Geometry check sheet. Reference: the model listing, model coordinates, mm. Face numbers are marked on the shaded views. A direction names the side the tool comes from. Round coordinates to 2 decimals unless told otherwise and drop trailing zeros. Write each loop counter-clockwise with the first axis right and the second up, starting at its lowest first coordinate (ties: lowest second). Pieces come first, ordered by that corner, then holes. Notation, with made-up numbers: M -11,38.25 L 10,38.25 A22 ccw 10,60.25 Z; hole C -22.5,-3.5 d8. An arc over 180 degrees is marked long. One line per item, written item: value. Start each with the question number.
1. Scan lines: probe 1 along Y at (x, z) = (2.5, -4.5); probe 2 along X at (y, z) = (7.25, 0); probe 3 along X at (y, z) = (21, 1). Record each from-to range of solid material in increasing order. Write a range as [from, to].
2. Access from +Z, -Z, +X, -X, +Y, -Y to the whole of each face (thin tool, end or side, straight path). Record for the marked faces 4, 5 and 6.
3. Section check C-C (z = -4.75). Record the boundary of the cut face in (x, y), and give its area (3 significant figures).
4. Release check for a two-part mould opening along X. For the marked faces 1, 2 and 3 record: pulls with the +X half, pulls with the -X half, needs draft (parallel to the pull), parting line crosses it, or undercut.
5. Section check B-B (x = 6). Record the boundary of the cut face in (y, z), and give its area (3 significant figures).
6. Depth check by flat-ended pin: P1, Ø4, axis at y = 17, z = -3.5, coming from the +X side; P2, Ø10, axis at x = 4, y = 8, coming from the +Z side; P3, Ø6, axis at x = 10.5, y = 8, coming from the +Z side. Enter the tip coordinate at first touch or a pass-through.
7. Section check D-D (y = 6.75). Record the boundary of the cut face in (x, z).
8. Section check A-A (x = 8.25). Record the boundary of the cut face in (y, z).
Autodesk Fusion 360 part; units mm, degrees
sketch "Sketch1" plane through (0, 0, 0) normal (0, 1, 0) x (1, 0, 0)
  line L0 (-6.9583, -4.2531) -> (13.0417, -4.2531)
  line L1 (13.0417, -4.2531) -> (13.0417, 8.7469)
  line L2 (13.0417, 8.7469) -> (-6.9583, 8.7469)
  line L3 (-6.9583, 8.7469) -> (-6.9583, -4.2531)
  line L4 (-6.9583, -4.2531) -> (1.0417, -4.2531)
  line L5 (1.0417, -4.2531) -> (1.0417, 8.7469)
  line L6 (1.0417, 8.7469) -> (-6.9583, 8.7469)
  line L7 (-6.9583, 8.7469) -> (-6.9583, -4.2531)
  dimension "d4" = 20
  dimension "d5" = 13
  dimension "d7" = 8
  dimension "d8" = 13
extrude "Extrude1" add sketch "Sketch1" along normal blind 23.5 contours L0 L2 L3 L4 L5 L6 L7
extrude "Extrude2" add sketch "Sketch1" along normal blind 3 contours L0 L1 L2 L5
sketch "Sketch2" plane through (1.0417, 0, 0) normal (1, 0, 0) x (0, 1, 0)
  line L0 (3, -8.7469) -> (23.5, -8.7469)
  line L1 (23.5, -8.7469) -> (23.5, 4.2531)
  line L2 (23.5, 4.2531) -> (3, 4.2531)
  line L3 (3, -0.2469) -> (18.5, -0.2469)
  line L4 (23.5, 4.2531) -> (18.4635, 4.2531)
  line L5 (18.4635, 4.2531) -> (18.4635, -8.7469)
  line L6 (18.4635, -8.7469) -> (23.5, -8.7469)
  line L7 (23.5, -8.7469) -> (23.5, 4.2531)
  line L8 (3, 4.2531) -> (3, -8.7469)
  dimension "d16" = 15.5
extrude "Extrude3" add sketch "Sketch2" along normal blind 12 contours L0 L1 L2 L4 L5 L6 L7
fillet "Fillet1" radius 2 1 edges at (-6.9583, 23.5, -2.2469)
fillet "Fillet2" radius 2 1 edges at (-6.9583, 0, -2.2469)
fillet "Fillet3" radius 1 1 edges at (13.0417, 18.4635, -2.2469)
fillet "Fillet4" radius 1 1 edges at (13.0417, 0, -2.2469)
sketch "Sketch3" plane through (0, 23.5, 0) normal (0, 1, 0) x (-1, 0, 0)
  line L0 (4.9583, -8.7469) -> (4.9583, 4.2531)
  line L1 (4.9583, 4.2531) -> (-13.0417, 4.2531)
  line L2 (-13.0417, 4.2531) -> (-13.0417, -8.7469)
  line L3 (-13.0417, -8.7469) -> (4.9583, -8.7469)
  line L4 (4.9583, -2.2469) -> (-13.0417, -2.2469)
  line L5 (-8.5241, 4.0524) -> (-8.5241, 0.8024)
  line L6 (-8.5417, -8.8028) -> (-8.5417, -5.5528)
  circle A0 centre (-8.5241, 0.8024) radius 1.3
  circle A1 centre (-8.5417, -5.5528) radius 1.3
  line L7 (-13.0417, 0.8028) -> (-8.5417, 0.8028)
  line L8 (-13.0417, -5.5528) -> (-8.5417, -5.5528)
  dimension "d32" = 3.25
  dimension "d33" = 3.25
  dimension "d34" = 2.6
  dimension "d35" = 2.6
  dimension "d36" = 4.5
  dimension "d37" = 4.5
hole "Hole2" at (8.5417, 23.5, 0.8028) at (8.5417, 23.5, -5.5528) direction (0, -1, 0) diameter 2.529 depth 10 tip angle 118
equation "clamp_w = 20 mm"
equation "clamp_l = 13 mm"
equation "clamp_bot_thickness = 3 mm"
equation "d4 = clamp_w"
equation "d5 = clamp_l"
equation "clamp_mid_w = 8 mm"
equation "d7 = clamp_mid_w"
equation "d8 = clamp_l"
equation "clamp_mid_thickness = deck_bed_gap + clamp_bot_thickness + clamp_top_thickness"
equation "d10 = clamp_mid_thickness"
equation "d12 = clamp_bot_thickness"
equation "clamp_top_thickness = 5 mm"
equation "deck_bed_gap = 15.5 mm"
equation "d16 = deck_bed_gap"
equation "top_clamp_depth = clamp_w - clamp_mid_w"
equation "d18 = top_clamp_depth"
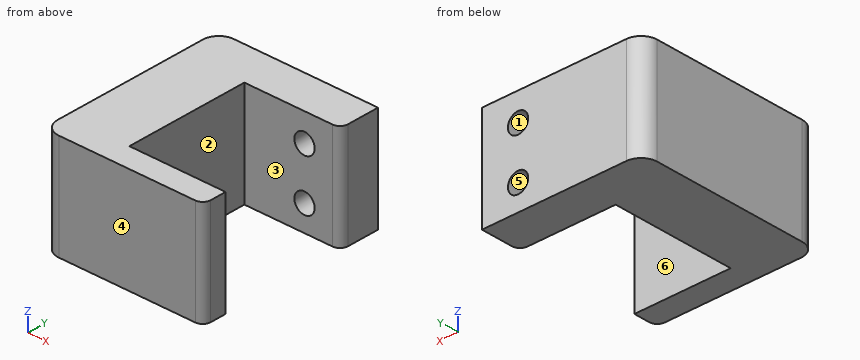
Result sheet:
1. probe 1: y = [0, 3], [18.46, 23.5]
1. probe 2: x = [-6.96, 1.04]
1. probe 3: x = [-6.96, 7.29], [9.79, 13.04]
2. face 4: +Z, -Z, +X, -X, -Y
2. face 5: +Y
2. face 6: +Z, -Z, +X
3. outline: M -6.96,2 A2 ccw -4.96,0 L 12.04,0 A1 ccw 13.04,1 L 13.04,3 L 1.04,3 L 1.04,18.46 L 7.56,18.46 L 7.56,23.5 L -4.96,23.5 A2 ccw -6.96,21.5 Z; M 9.52,18.46 L 12.04,18.46 A1 ccw 13.04,19.46 L 13.04,23.5 L 9.52,23.5 Z
3. area: 272 mm2
4. face 1: undercut
4. face 2: pulls with the +X half
4. face 3: needs draft
5. outline: M 0,-8.75 L 3,-8.75 L 3,4.25 L 0,4.25 Z; M 18.46,-8.75 L 23.5,-8.75 L 23.5,4.25 L 18.46,4.25 Z
5. area: 104 mm2
6. P1: stops at x = 12.93
6. P2: stops at z = 4.25
6. P3: passes through
7. outline: M -6.96,-8.75 L 1.04,-8.75 L 1.04,4.25 L -6.96,4.25 Z
8. outline: M 0,-8.75 L 3,-8.75 L 3,4.25 L 0,4.25 Z; M 18.46,-8.75 L 23.5,-8.75 L 23.5,-6.78 L 18.46,-6.78 Z; M 18.46,-4.32 L 23.5,-4.32 L 23.5,-0.43 L 18.46,-0.43 Z; M 18.46,2.03 L 23.5,2.03 L 23.5,4.25 L 18.46,4.25 Z
